```python
from build123d import *

# Parameters (mm, degrees)
SKETCH_2_W          = 24.2
SKETCH_2_H          = 24.2
SKETCH_2_W_2        = 20.2
SKETCH_2_H_2        = 20.2
EXTRUDE_4_DEPTH     = 100
SKETCH_6_W          = 24.2
SKETCH_6_H          = 24.2
SKETCH_6_W_2        = 20.2
SKETCH_6_H_2        = 20.2
EXTRUDE_5_DEPTH     = 40
SKETCH_7_R          = 2.5
CUT_EXTRUDE_1_DEPTH = 40
SKETCH_8_R          = 2.5
CUT_EXTRUDE_2_DEPTH = 40
CUT_EXTRUDE_START   = -40
SKETCH_9_W          = 20
SKETCH_9_H          = 24.2
SKETCH_9_R          = 2.5
CUT_EXTRUDE_3_DEPTH = 40
SKETCH_10_W         = 24.2
SKETCH_10_H         = 20
SKETCH_10_R         = 2.5
CUT_EXTRUDE_4_DEPTH = 40
SKETCH_11_W         = 69.821202151
SKETCH_11_H         = 48.665955669
CUT_EXTRUDE_5_DEPTH = 12.1
SKETCH_12_W         = 20.2
SKETCH_12_H         = 2
CUT_EXTRUDE_6_DEPTH = 10
SKETCH_13_W         = 20.2
SKETCH_13_H         = 2
CUT_EXTRUDE_7_DEPTH = 0.1
FILLET_1_R          = 5
FILLET_2_R          = 5


with BuildPart() as part:
    # 草图2 → 凸台-拉伸4 (new body)
    with BuildSketch(Plane.XY):
        Rectangle(SKETCH_2_W, SKETCH_2_H)
        Rectangle(SKETCH_2_W_2, SKETCH_2_H_2, mode=Mode.SUBTRACT)
    extrude(amount=EXTRUDE_4_DEPTH)

    # 草图6 → 凸台-拉伸5 (add)
    with BuildSketch(Plane(origin=(0, 12.1, 0), x_dir=(1, 0, 0), z_dir=(0, 1, 0))):
        with Locations((0, -50)):
            Rectangle(SKETCH_6_W, SKETCH_6_H)
        with Locations((0, -50)):
            Rectangle(SKETCH_6_W_2, SKETCH_6_H_2, mode=Mode.SUBTRACT)
    extrude(amount=EXTRUDE_5_DEPTH)

    # 草图7 → 切除-拉伸1 (cut)
    with BuildSketch(Plane.ZY.offset(12.1)):
        with Locations((10, 0)):
            Circle(SKETCH_7_R)
        with Locations((30, 0)):
            Circle(SKETCH_7_R)
        with Locations(Location((90, 0, 0), (0, 0, 180))):
            Circle(SKETCH_7_R)
        with Locations(Location((70, 0, 0), (0, 0, 180))):
            Circle(SKETCH_7_R)
        with Locations((50, 42.1)):
            Circle(SKETCH_7_R)
        with Locations((50, 22.1)):
            Circle(SKETCH_7_R)
    extrude(amount=-CUT_EXTRUDE_1_DEPTH, mode=Mode.SUBTRACT)

    # 草图8 → 切除-拉伸2 (cut)
    with BuildSketch(Plane(origin=(12.1, 0, 0), x_dir=(0, 0, -1), z_dir=(1, 0, 0))):
        with Locations((-50, 0)):
            Circle(SKETCH_8_R)
    extrude(amount=-CUT_EXTRUDE_2_DEPTH, mode=Mode.SUBTRACT)

    # 草图9 → 切除-拉伸3 (cut)
    # profile 1 of 2: a face of its own
    with BuildSketch(Plane(origin=(12.1, 0, 0), x_dir=(0, 0, -1), z_dir=(1, 0, 0)).offset(CUT_EXTRUDE_START)):
        with Locations((-10, 0)):
            Rectangle(SKETCH_9_W, SKETCH_9_H)
        with Locations((-10, 0)):
            Circle(SKETCH_9_R, mode=Mode.SUBTRACT)
    # profile 2 of 2: a face of its own
    with BuildSketch(Plane(origin=(12.1, 0, 0), x_dir=(0, 0, -1), z_dir=(1, 0, 0)).offset(CUT_EXTRUDE_START)):
        with Locations((-90, 0)):
            Rectangle(SKETCH_9_W, SKETCH_9_H)
        with Locations((-90, 0)):
            Circle(SKETCH_9_R, mode=Mode.SUBTRACT)
    extrude(amount=CUT_EXTRUDE_3_DEPTH, mode=Mode.SUBTRACT)

    # 草图10 → 切除-拉伸4 (cut)
    with BuildSketch(Plane(origin=(12.1, 0, 0), x_dir=(0, 0, -1), z_dir=(1, 0, 0)).offset(CUT_EXTRUDE_START)):
        with Locations((-50, 42.1)):
            Rectangle(SKETCH_10_W, SKETCH_10_H)
        with Locations((-50, 42.1)):
            Circle(SKETCH_10_R, mode=Mode.SUBTRACT)
    extrude(amount=CUT_EXTRUDE_4_DEPTH, mode=Mode.SUBTRACT)

    # 草图11 → 切除-拉伸5 (cut)
    with BuildSketch(Plane(origin=(12.1, 0, 0), x_dir=(0, 0, -1), z_dir=(1, 0, 0))):
        with Locations((-50.999985391, 8.600020454)):
            Rectangle(SKETCH_11_W, SKETCH_11_H)
    extrude(amount=-CUT_EXTRUDE_5_DEPTH, mode=Mode.SUBTRACT)

    # 草图12 → 切除-拉伸6 (cut)
    with BuildSketch(Plane(origin=(0, 0, 0), x_dir=(0, 0, -1), z_dir=(1, 0, 0))):
        with Locations((-50, 11.1)):
            Rectangle(SKETCH_12_W, SKETCH_12_H)
    extrude(amount=-CUT_EXTRUDE_6_DEPTH, mode=Mode.SUBTRACT)

    # 草图13 → 切除-拉伸7 (cut)
    with BuildSketch(Plane(origin=(-10, 0, 0), x_dir=(0, 0, -1), z_dir=(1, 0, 0))):
        with Locations((-50, 11.1)):
            Rectangle(SKETCH_13_W, SKETCH_13_H)
    extrude(amount=-CUT_EXTRUDE_7_DEPTH, mode=Mode.SUBTRACT)

    # 圆角1
    fillet_1_edges = [part.edges().sort_by_distance(p)[0] for p in [
        (-6.05, 12.1, 37.9),
    ]]
    fillet(fillet_1_edges, radius=FILLET_1_R)

    # 圆角2
    fillet_2_edges = [part.edges().sort_by_distance(p)[0] for p in [
        (-6.05, 12.1, 62.1),
    ]]
    fillet(fillet_2_edges, radius=FILLET_2_R)


solid = part.part
```
Model file for the job. Use its own axes, mm. A direction names the side the tool comes from. Round coordinates to 2 decimals unless told otherwise and drop trailing zeros. Loops run counter-clockwise (first coordinate to the right, second up) from the corner with the lowest first, then second, coordinate; pieces in that order, holes last. Notation, with made-up numbers: M 86,25.25 L 127,25.25 A12 ccw 127,48.25 Z; hole C 23,-29 d11. An arc over 180 degrees is marked long. Put each result on its own line as item: value. Start each with the question number.
Item 1: Mould opens along Y. For faces 1 (the face through (-5, 21, 39.9)), 2 (the face through (-6, 12.1, 73)), 3 (the face through (-11.11, 21.14, 52.31)) say: released by +Y, released by -Y, zero draft, split by the parting line, or undercut.
Item 2: Drill centre lines: line 1 along Y through (x, z) = (-10.8, 50); line 2 along Y through (x, z) = (-4.5, 32); line 3 along Y through (x, z) = (-10.7, 70). Where is each one in solid material? Low to high.
Item 3: Cut at C-C (x = -4.75). List the corners of the cut face in (y, z).
Item 4: 3-axis set-ups, long thin cutter, end or side, ignore diameter. For faces 4 (the face through (-6, 24, 62.1)), 5 (the face through (-6, 12.1, 26)), 6 (the face through (-5, 10.1, 70)): which of +Z, -Z, +X, -X, +Y, -Y reach the whole face in a straight line?
Item 5: Cut at D-D (z = 70). List the corners of the cut face in (x, y).
Item 6: Cut at A-A (y = 22.1). List the corners of the cut face in (x, z).
Item 7: Cut at B-B (z = 50). List the corners of the cut face in (x, y), then the cut area to 3 significant figures.
Item 8: Drop flat-ended pins along their axis: P1, Ø6, axis at y = 0, z = 50, coming from the +X side; P2, Ø6, axis at x = -8.5, y = -6.5, coming from the +Z side; P3, Ø1, axis at x = -8.5, y = -4.5, coming from the -Z side; P4, Ø3.5, axis at x = -8, z = 27.5, coming from the +Y side. Give the stop position or say it passes through.
Answer block:
1. face 1: zero draft
1. face 2: released by +Y
1. face 3: undercut
2. line 1: -12.1 to -2.5, 2.5 to 19.6, 24.6 to 32.1
2. line 2: -12.1 to -10.1, 10.1 to 12.1
2. line 3: -12.1 to -2.5, 2.5 to 12.1
3. outline: M -12.1,20 L -10.1,20 L -10.1,80 L -12.1,80 Z; M 10.1,20 L 12.1,20 L 12.1,32.9 A5 cw 17.1,37.9 L 32.1,37.9 L 32.1,39.9 L 10.1,39.9 Z; M 10.1,60.1 L 32.1,60.1 L 32.1,62.1 L 17.1,62.1 A5 cw 12.1,67.1 L 12.1,80 L 10.1,80 Z
4. face 4: +Z, +X, -X, +Y
4. face 5: -Z, +X, -X, +Y
4. face 6: +Z, -Z, +X
5. outline: M -12.1,-12.1 L 0,-12.1 L 0,-10.1 L -10.1,-10.1 L -10.1,-2.5 L -12.1,-2.5 Z; M -12.1,2.5 L -10.1,2.5 L -10.1,10.1 L 0,10.1 L 0,12.1 L -12.1,12.1 Z
6. outline: M -12.1,37.9 L 0,37.9 L 0,39.9 L -10.1,39.9 L -10.1,47.5 L -12.1,47.5 Z; M -12.1,52.5 L -10.1,52.5 L -10.1,60.1 L 0,60.1 L 0,62.1 L -12.1,62.1 Z
7. outline: M -12.1,-12.1 L 0,-12.1 L 0,-10.1 L -10.1,-10.1 L -10.1,-2.5 L -12.1,-2.5 Z; M -12.1,2.5 L -10.1,2.5 L -10.1,19.6 L -12.1,19.6 Z; M -12.1,24.6 L -10.1,24.6 L -10.1,32.1 L -12.1,32.1 Z
7. area: 88.6 mm2
8. P1: x = -10.1
8. P2: z = 80
8. P3: through
8. P4: y = 12.1
